Design review of the part shown in the three views and the two pictorial views. Dimensions are in mm from the part's minimum x, y and z. Give positions to 0.01 mm unless a question says otherwise; leave off trailing zeros. Order: outer loops, then holes, each group sorted by start corner. A loop starts at its lowest first (then second) coordinate and runs counter-clockwise, first axis right, second up. Notation, with made-up numbers: M 77,-14.5 L 117,-14.5 A16 ccw 117,14.5 Z; hole C -13,70.25 d5. An arc over 180 degrees is marked long. Answer as a JSON object with one key per item and string values.
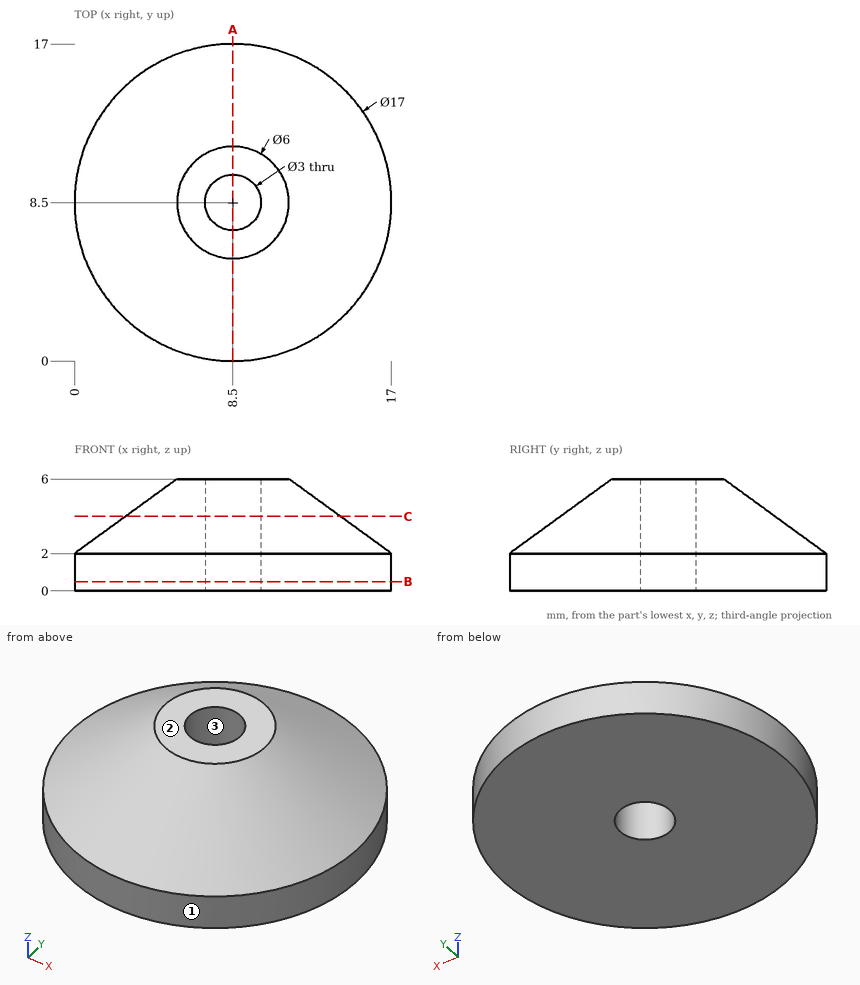
(1) We need section B-B (z = 0.5). Write out the cut boundary in (x, y), plus the area to 3 significant figures.
Checked values:
{"outline": "C 8.5,8.5 d17; hole C 8.5,8.5 d3", "area": "220 mm^2"}
(2) To check wall thickness, follow L1, parallel to X at y = 9.75, z = 1; L2, parallel to X at y = 8.75, z = 2.5; L3, parallel to Y at x = 7.5, z = 1.5. State the ranges of each line that lie inside material, in increasing order. Write a range as from..to.
Checked values:
{"L1": "x = 0.09..7.67, 9.33..16.91", "L2": "x = 0.69..7.02, 9.98..16.31", "L3": "y = 0.06..7.38, 9.62..16.94"}
(3) We need section C-C (z = 4). Write out the cut boundary in (x, y), plus the area to 3 significant figures.
Checked values:
{"outline": "C 8.5,8.5 d11.5; hole C 8.5,8.5 d3", "area": "96.8 mm^2"}
(4) Draft analysis for pull direction Y (two halves, no side actions). For the marked faces 1, 2 and 3, state which applies: +Y half, -Y half, draft (parallel to the pull), parting line (faces both ways), or undercut.
Checked values:
{"face 1": "parting line", "face 2": "draft", "face 3": "undercut"}
(5) Insertion check: pin 1 (2.5 mm diameter, centred on x = 8.5, y = 8.5, fed in from +Z); pin 2 (3 mm diameter, centred on x = 14, z = 4, fed in from +Y); pin 3 (2 mm diameter, centred on x = 12.5, z = 5, fed in from +Y). Each pin has a flat end and moves straight along its axis. Give the tip position at first contact, or say it passes through.
Checked values:
{"pin 1": "passes through", "pin 2": "stops at y = 14.36", "pin 3": "stops at y = 12.84"}
(6) We need section A-A (x = 8.5). Write out the cut boundary in (y, z), plus the area to 3 significant figures.
Checked values:
{"outline": "M 0,0 L 7,0 L 7,6 L 5.5,6 L 0,2 Z; M 10,0 L 17,0 L 17,2 L 11.5,6 L 10,6 Z", "area": "62.0 mm^2"}
